Read the model definition and answer for the solid it produces. Units are mm, in the model's axes. Face numbers are marked on the shaded views. A direction names the side the tool comes from. Coordinates: 2 decimals unless noted, no trailing zeros. Write each loop counter-clockwise with the first axis right and the second up, starting at its lowest first coordinate (ties: lowest second). Pieces come first, ordered by that corner, then holes.
Item 1: Section A-A (x = 36.5) is taken. Give the vertices of the cut face in (y, z).
Item 2: A tool of negligible diameter and unlimited length cuts with its end or side. For the marked faces 4, 5 and 6, from which of +Z, -Z, +X, -X, +Y, -Y can it reach the whole face along a straight path? Write none if from no direction.
Item 3: Determine the mould class of the marked faces 1, 2 and 3 for opening direction Y: released by +Y, released by -Y, zero draft, split by the parting line, or undercut.
Item 4: Section D-D (y = 11.5) is taken. Give the vertices of the cut face in (x, z), then the cut area to 3 significant figures.
Item 5: Each of these flat-tipped pins is pushed along its axis until it touches: P1, Ø6, axis at x = -13.5, z = 3, coming from the -Y side; P2, Ø6, axis at x = 17.53, y = -17.53, coming from the +Z side; P3, Ø5, axis at x = 26.5, y = -1, coming from the +Z side; P4, Ø6, axis at y = 20, z = -7, coming from the -X side. Where does it stop, or does it pass through?
Item 6: Section C-C (z = 1) is taken. State how many separate pieces and enclosed holes the cut face has, then the cut area to 3 significant figures.
Item 7: Straight lines are drawn through the part: probe 1 along Y at (x, z) = (0, -5.25); probe 2 along Y at (x, z) = (-18.5, -6.25); probe 3 along X at (y, z) = (-0.5, -6). For each, find the intervals that lie inside material, in ascending order.
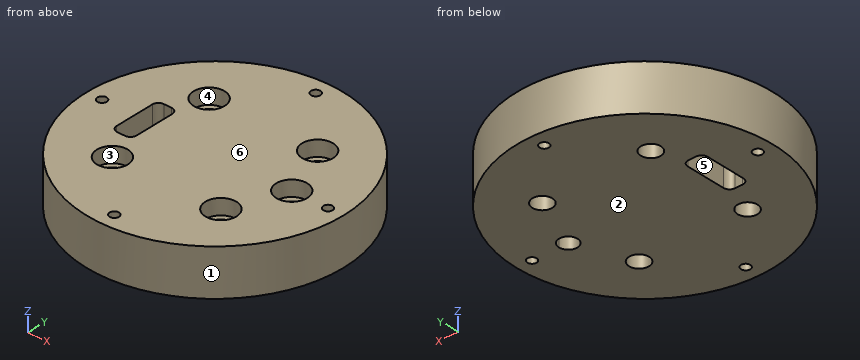
from build123d import *

# Parameters (mm, degrees)
SKETCH_1_R           = 41.5
EXTRUDE_1_DEPTH      = 5
EXTRUDE_1_DEPTH_BACK = 10
SKETCH_2_R           = 5
CUT_EXTRUDE_1_DEPTH  = 5
SKETCH_4_R           = 1.5
CUT_EXTRUDE_2_DEPTH  = 16


with BuildPart() as part:
    # 草图1 → 凸台-拉伸1 (new body, two sides)
    with BuildSketch(Plane.XY) as extrude_1_sk:
        Circle(SKETCH_1_R)
        with BuildLine():
            ThreePointArc((-20.75113276, -17.528548354), (-17.528548354, -14.305963949), (-14.305963949, -17.528548354))
            ThreePointArc((-14.305963949, -17.528548354), (-17.528548354, -20.75113276), (-20.75113276, -17.528548354))
        make_face(mode=Mode.SUBTRACT)
        with BuildLine():
            ThreePointArc((14.305963949, -17.528548354), (17.528548354, -14.305963949), (20.75113276, -17.528548354))
            ThreePointArc((20.75113276, -17.528548354), (17.528548354, -20.75113276), (14.305963949, -17.528548354))
        make_face(mode=Mode.SUBTRACT)
        with BuildLine():
            Line((-24.045437487, 8.428297676), (-21.566526406, 8.428297676))
            ThreePointArc((-21.566526406, 8.428297676), (-20.68362959, 8.220920288), (-19.985383241, 7.642159365))
            ThreePointArc((-19.985383241, 7.642159365), (-19.686578169, 7.076512396), (-19.583397541, 6.445168811))
            Line((-19.583397541, 6.445168811), (-19.583397541, -6.445168811))
            ThreePointArc((-19.583397541, -6.445168811), (-20.164242538, -7.847452679), (-21.566526406, -8.428297676))
            Line((-21.566526406, -8.428297676), (-24.045437487, -8.428297676))
            ThreePointArc((-24.045437487, -8.428297676), (-25.447721356, -7.847452679), (-26.028566352, -6.445168811))
            Line((-26.028566352, -6.445168811), (-26.028566352, 6.445168811))
            ThreePointArc((-26.028566352, 6.445168811), (-25.447721356, 7.847452679), (-24.045437487, 8.428297676))
        make_face(mode=Mode.SUBTRACT)
        with BuildLine():
            ThreePointArc((-20.75113276, 17.528548354), (-17.528548354, 20.75113276), (-14.305963949, 17.528548354))
            ThreePointArc((-14.305963949, 17.528548354), (-17.528548354, 14.305963949), (-20.75113276, 17.528548354))
        make_face(mode=Mode.SUBTRACT)
        with BuildLine():
            ThreePointArc((14.305963949, 17.528548354), (17.528548354, 20.75113276), (20.75113276, 17.528548354))
            ThreePointArc((20.75113276, 17.528548354), (17.528548354, 14.305963949), (14.305963949, 17.528548354))
        make_face(mode=Mode.SUBTRACT)
        with BuildLine():
            ThreePointArc((21.814417514, 0), (24.789110812, 2.974693297), (27.763804109, 0))
            ThreePointArc((27.763804109, 0), (24.789110812, -2.974693297), (21.814417514, 0))
        make_face(mode=Mode.SUBTRACT)
    extrude(amount=EXTRUDE_1_DEPTH)
    extrude(extrude_1_sk.sketch, amount=-EXTRUDE_1_DEPTH_BACK)

    # 草图2 → 切除-拉伸1 (cut)
    with BuildSketch(Plane.XY.offset(5)):
        with Locations((-17.528548354, 17.528548354)):
            Circle(SKETCH_2_R)
        with BuildLine():
            ThreePointArc((-20.75113276, 17.528548354), (-17.528548354, 14.305963949), (-14.305963949, 17.528548354))
            ThreePointArc((-14.305963949, 17.528548354), (-17.528548354, 20.75113276), (-20.75113276, 17.528548354))
        make_face(mode=Mode.SUBTRACT)
        with Locations((17.528548354, 17.528548354)):
            Circle(SKETCH_2_R)
        with BuildLine():
            ThreePointArc((20.75113276, 17.528548354), (17.528548354, 20.75113276), (14.305963949, 17.528548354))
            ThreePointArc((14.305963949, 17.528548354), (17.528548354, 14.305963949), (20.75113276, 17.528548354))
        make_face(mode=Mode.SUBTRACT)
        with Locations((-17.528548354, -17.528548354)):
            Circle(SKETCH_2_R)
        with BuildLine():
            ThreePointArc((-20.75113276, -17.528548354), (-17.528548354, -20.75113276), (-14.305963949, -17.528548354))
            ThreePointArc((-14.305963949, -17.528548354), (-17.528548354, -14.305963949), (-20.75113276, -17.528548354))
        make_face(mode=Mode.SUBTRACT)
        with Locations((17.528548354, -17.528548354)):
            Circle(SKETCH_2_R)
        with BuildLine():
            ThreePointArc((14.305963949, -17.528548354), (17.528548354, -20.75113276), (20.75113276, -17.528548354))
            ThreePointArc((20.75113276, -17.528548354), (17.528548354, -14.305963949), (14.305963949, -17.528548354))
        make_face(mode=Mode.SUBTRACT)
        with Locations((24.789110812, 0)):
            Circle(SKETCH_2_R)
        with BuildLine():
            ThreePointArc((21.814417514, 0), (24.789110812, -2.974693297), (27.763804109, 0))
            ThreePointArc((27.763804109, 0), (24.789110812, 2.974693297), (21.814417514, 0))
        make_face(mode=Mode.SUBTRACT)
    extrude(amount=-CUT_EXTRUDE_1_DEPTH, mode=Mode.SUBTRACT)

    # 草图4 → 切除-拉伸2 (cut, through all)
    with BuildSketch(Plane.XY.offset(5)):
        with Locations((-36.5, 0)):
            Circle(SKETCH_4_R)
        with Locations((0, -36.5)):
            Circle(SKETCH_4_R)
        with Locations((36.5, 0)):
            Circle(SKETCH_4_R)
        with Locations((0, 36.5)):
            Circle(SKETCH_4_R)
    extrude(amount=-CUT_EXTRUDE_2_DEPTH, mode=Mode.SUBTRACT)


solid = part.part
Established:
1. outline: (-19.75, -10) - (-1.5, -10) - (-1.5, 5) - (-19.75, 5) - close; (1.5, -10) - (19.75, -10) - (19.75, 5) - (1.5, 5) - close
2. face 4: +Z
2. face 5: +Z, -Z
2. face 6: +Z, +X, -X, +Y, -Y
3. face 1: split by the parting line
3. face 2: zero draft
3. face 3: undercut
4. outline: (-39.87, -10) - (39.87, -10) - (39.87, 5) - (-39.87, 5) - close
4. area: 1,200 mm2
5. P1: stops at y = -40.15
5. P2: passes through
5. P3: stops at z = 0
5. P4: stops at x = -37.86
6. separate pieces: 1
6. enclosed holes: 10
6. area: 4,880 mm2
7. probe 1: y = -41.5 to -38, -35 to 35, 38 to 41.5
7. probe 2: y = -37.15 to -20.6, -14.46 to 14.46, 20.6 to 37.15
7. probe 3: x = -41.5 to -37.91, -35.09 to -26.03, -19.58 to 21.86, 27.72 to 35.09, 37.91 to 41.5
